Input: dimensioned drawing with shaded views. Units: mm. Origin: part minimum x, y, z. A direction names the side the tool comes from. Give positions to 0.01 mm unless a question says otherwise; leave off trailing zeros. Write each loop counter-clockwise with the first axis right and the second up, starting at its lowest first coordinate (ties: lowest second). Pieces come first, ordered by that corner, then holes. Notation, with made-up numbers: (85.25, -3.75) -> (121.25, -3.75) arc R28 ccw to (121.25, 33.25) -> close; hole circle Ø10 at (1, -23.5). An arc over 180 degrees is marked (long way). Return JSON: item names as keys, results as strings. Group by question number.
Item 1: Section B-B, the plane z = 8. Return loops of the section in (x, y).
Item 2: Line query: line 1 (Y direction, x = 85, z = 6); line 2 (Y direction, x = 40, z = 16); line 3 (X direction, y = 40, z = 10). Output: solid intervals per line, ascending. Write a range as [from, to].
Item 3: Section D-D, the plane y = 44. Return loops of the section in (x, z) (1 decimal).
Item 4: Section C-C, the plane x = 71. Return loops of the section in (y, z), then the cut area to 3 significant figures.
Item 5: Mould query, pull axis X, two halves, no side actions, for the marked faces 5, 6 and 7. Classes: released by +X, released by -X, zero draft, split by the parting line, or undercut.
Item 6: Set-up query: the marked faces 1, 2, 3 and 4. Return all of +Z, -Z, +X, -X, +Y, -Y with unobstructed straight access to the full face (end or side cutting, diameter ignored); none if empty.
Item 7: Section A-A, the plane y = 13. Return loops of the section in (x, z), then the cut area to 4 significant figures.
Item 8: Pin query (flat end, axial travel): P1, Ø8, axis at x = 85, y = 40, coming from the -Z side (1 decimal); P2, Ø10, axis at y = 34, z = 26, coming from the -X side; P3, Ø12, axis at y = 24.5, z = 4, coming from the -X side; P4, Ø13, axis at x = 40, y = 25, coming from the +Z side. Return the tip coordinate at first contact, or that it passes through.
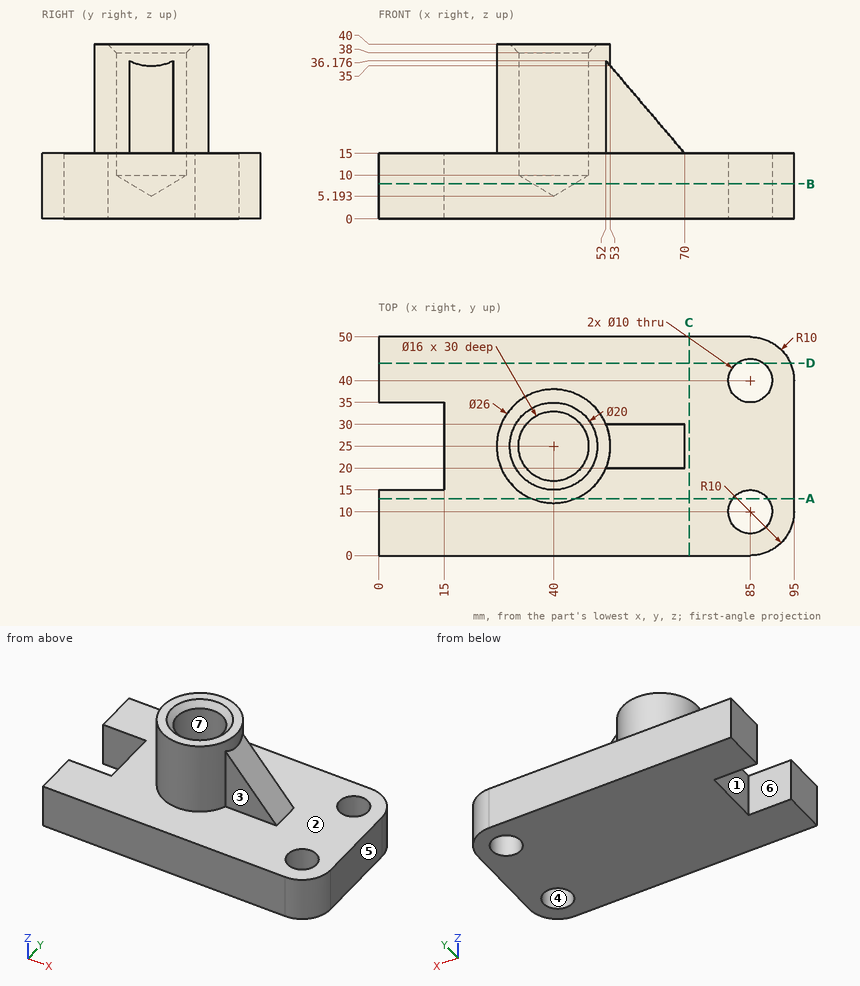
Answer below:
{
 "1": {"outline": "(0, 0) -> (85, 0) arc R10 ccw to (95, 10) -> (95, 40) arc R10 ccw to (85, 50) -> (0, 50) -> (0, 35) -> (15, 35) -> (15, 15) -> (0, 15) -> close; hole circle Ø9.34 at (40, 25); hole circle Ø10 at (85, 10); hole circle Ø10 at (85, 40)"},
 "2": {"line 1": "y = [0, 5], [15, 35], [45, 50]", "line 2": "y = [12, 17], [33, 38]", "line 3": "x = [0, 80], [90, 95]"},
 "3": {"outline": "(0, 0) -> (82, 0) -> (82, 15) -> (0, 15) -> close; (88, 0) -> (94.2, 0) -> (94.2, 15) -> (88, 15) -> close"},
 "4": {"outline": "(0, 0) -> (50, 0) -> (50, 15) -> (0, 15) -> close", "area": "750 mm2"},
 "5": {"face 5": "released by +X", "face 6": "zero draft", "face 7": "undercut"},
 "6": {"face 1": "+Z, -Z, -X", "face 2": "+Z", "face 3": "+Z, +X, -Y", "face 4": "+Z, -Z"},
 "7": {"outline": "(0, 0) -> (81, 0) -> (81, 15) -> (45, 15) -> (45, 40) -> (35, 40) -> (35, 15) -> (0, 15) -> close; (89, 0) -> (95, 0) -> (95, 15) -> (89, 15) -> close", "area": "1,555 mm2"},
 "8": {"P1": "passes through", "P2": "stops at x = 27.63", "P3": "stops at x = 15", "P4": "stops at z = 9.1"}
}
